Design review of the part shown in the three views and the two pictorial views. Dimensions are in mm from the part's minimum x, y and z. A direction names the side the tool comes from. Round coordinates to 2 decimals unless told otherwise and drop trailing zeros. Order: outer loops, then holes, each group sorted by start corner. A loop starts at its lowest first (then second) coordinate and runs counter-clockwise, first axis right, second up. Notation, with made-up numbers: (43, 38.25) - (67, 38.25) arc R16 ccw to (67, 68.25) - close; hole circle Ø4 at (73.5, 49). An arc over 180 degrees is marked (long way). Use CSV: the item, a comma, the result in double quotes.
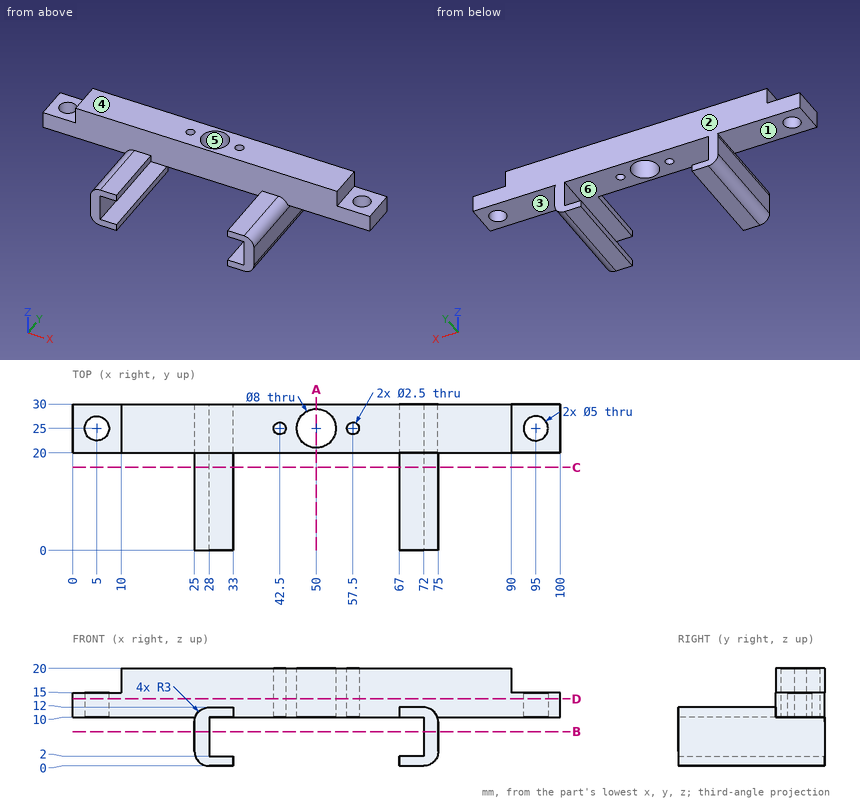
1) We need section D-D (z = 13.75). Give the boundary of the cut face in (x, y), then the cut area to 3 significant figures.
Data:
outline,"(0, 20) - (100, 20) - (100, 30) - (0, 30) - close; hole circle Ø5 at (5, 25); hole circle Ø2.5 at (42.5, 25); hole circle Ø8 at (50, 25); hole circle Ø2.5 at (57.5, 25); hole circle Ø5 at (95, 25)"
area,"901 mm2"
2) We need section C-C (y = 17). Give the boundary of the cut face in (x, z), then the cut area to 3 significant figures.
Data:
outline,"(25, 3) arc R3 ccw to (28, 0) - (33, 0) - (33, 2) - (28, 2) - (28, 10) - (33, 10) - (33, 12) - (28, 12) arc R3 ccw to (25, 9) - close; (67, 0) - (72, 0) arc R3 ccw to (75, 3) - (75, 9) arc R3 ccw to (72, 12) - (67, 12) - (67, 10) - (72, 10) - (72, 2) - (67, 2) - close"
area,"104 mm2"
3) Insertion check: pin 1 Ø5.5 at (x, y) = (68.5, 10.5) entering from +Z; pin 2 Ø1.6 at (y, z) = (15.5, 1.5) entering from +X; pin 3 Ø12 at (x, y) = (79, 6) entering from +Z. Each pin has a flat end and moves straight along its axis. Give the tip position at first contact, or say it passes through.
Data:
pin 1,"stops at z = 12"
pin 2,"stops at x = 74.92"
pin 3,"stops at z = 11.83"
4) For the marked faces 1, 2 and 3, list the 3-axis set-ups (+Z, -Z, +X, -X, +Y, -Y) from which the entire face can be reached by the end or side of a thin tool; tool diameter is ignored.
Data:
face 1,"-Z, -X, +Y, -Y"
face 2,"+Z, -Z, +X, -X, +Y"
face 3,"-Z, +X, +Y, -Y"
5) We need section B-B (z = 7). Give the boundary of the cut face in (x, y).
Data:
outline,"(25, 0) - (28, 0) - (28, 30) - (25, 30) - close; (72, 0) - (75, 0) - (75, 30) - (72, 30) - close"
6) The part is to be moulded in two halves that separate along X. For the marked faces 4, 5 and 6, say which applies: +X half, -X half, draft (parallel to the pull), parting line (faces both ways), or undercut.
Data:
face 4,"draft"
face 5,"undercut"
face 6,"undercut"
7) To check wall thickness, follow L1, parallel to X at y = 7.75, z = 6; L2, parallel to Y at x = 42.5, z = 17; L3, parallel to Z at x = 32, y = 10.75. State the ranges of each line that lie inside material, in increasing order. Write a range as from..to.
Data:
L1,"x = 25..28, 72..75"
L2,"y = 20..23.75, 26.25..30"
L3,"z = 0..2, 10..12"
8) We need section A-A (x = 50). Give the boundary of the cut face in (y, z), then the cut area to 3 significant figures.
Data:
outline,"(20, 10) - (21, 10) - (21, 20) - (20, 20) - close; (29, 10) - (30, 10) - (30, 20) - (29, 20) - close"
area,"20.0 mm2"
